Could you check a few things on this model? Use its own coordinates, in mm. A direction names the side the tool comes from. Round coordinates to 2 decimals unless told otherwise and drop trailing zeros. Write each loop counter-clockwise with the first axis right and the second up, starting at its lowest first coordinate (ties: lowest second). Pieces come first, ordered by that corner, then holes. Notation, with made-up numbers: (-14.5, 81) -> (20.5, 81) arc R36 cw to (20.5, 120) -> close; hole circle Ø11 at (80.5, -18.5). An arc over 180 degrees is marked (long way). Answer in a Markdown table with one row per item. Add a question column.
```python
from build123d import *

# Parameters (mm, degrees)
SKETCH1_W           = 31.75
SKETCH1_H           = 3.175
SKETCH1_W_2         = 3.175
SKETCH1_H_2         = 28.575
BOSS_EXTRUDE1_DEPTH = 19.05
SWITCH_MOUNT_REACH  = 5.175
SKETCH2_R           = 1.190625
SKETCH2_W           = 2.54
SKETCH2_H           = 0.254
BRACKET_MOUNT_REACH = 5.175
SKETCH3_R           = 3.175


with BuildPart() as part:
    # Sketch1 → Boss-Extrude1 (new body)
    with BuildSketch(Plane.XY):
        with Locations((-15.875, 1.5875)):
            Rectangle(SKETCH1_W, SKETCH1_H)
        with Locations((-1.5875, -14.2875)):
            Rectangle(SKETCH1_W_2, SKETCH1_H_2)
    extrude(amount=BOSS_EXTRUDE1_DEPTH)

    # Sketch2 → Switch Mount (cut, up to next)
    with BuildSketch(Plane.ZY.offset(3.175), mode=Mode.PRIVATE) as switch_mount_sk1:
        with Locations((4.318, -10.668)):
            Circle(SKETCH2_R)
    switch_mount_tool1 = extrude(switch_mount_sk1.sketch, amount=-SWITCH_MOUNT_REACH, mode=Mode.PRIVATE) & part.part
    add(switch_mount_tool1.solids().sort_by_distance((-3.175, -10.668, 4.318))[0], mode=Mode.SUBTRACT)
    # Sketch2 → Switch Mount (cut, up to next)
    with BuildSketch(Plane.ZY.offset(3.175), mode=Mode.PRIVATE) as switch_mount_sk2:
        with Locations((4.318, -20.193)):
            Circle(SKETCH2_R)
    switch_mount_tool2 = extrude(switch_mount_sk2.sketch, amount=-SWITCH_MOUNT_REACH, mode=Mode.PRIVATE) & part.part
    add(switch_mount_tool2.solids().sort_by_distance((-3.175, -20.193, 4.318))[0], mode=Mode.SUBTRACT)
    # Sketch2 → Switch Mount (cut, up to next)
    with BuildSketch(Plane.ZY.offset(3.175), mode=Mode.PRIVATE) as switch_mount_sk3:
        with Locations((1.27, -25.2222)):
            Rectangle(SKETCH2_W, SKETCH2_H)
    switch_mount_tool3 = extrude(switch_mount_sk3.sketch, amount=-SWITCH_MOUNT_REACH, mode=Mode.PRIVATE) & part.part
    add(switch_mount_tool3.solids().sort_by_distance((-3.175, -25.2222, 1.27))[0], mode=Mode.SUBTRACT)

    # Sketch3 → Bracket Mount (cut, up to next)
    with BuildSketch(Plane.XZ, mode=Mode.PRIVATE) as bracket_mount_sk1:
        with Locations((-9.525, 12.065)):
            Circle(SKETCH3_R)
    bracket_mount_tool1 = extrude(bracket_mount_sk1.sketch, amount=-BRACKET_MOUNT_REACH, mode=Mode.PRIVATE) & part.part
    add(bracket_mount_tool1.solids().sort_by_distance((-9.525, 0, 12.065))[0], mode=Mode.SUBTRACT)
    # Sketch3 → Bracket Mount (cut, up to next)
    with BuildSketch(Plane.XZ, mode=Mode.PRIVATE) as bracket_mount_sk2:
        with Locations((-22.225, 12.065)):
            Circle(SKETCH3_R)
    bracket_mount_tool2 = extrude(bracket_mount_sk2.sketch, amount=-BRACKET_MOUNT_REACH, mode=Mode.PRIVATE) & part.part
    add(bracket_mount_tool2.solids().sort_by_distance((-22.225, 0, 12.065))[0], mode=Mode.SUBTRACT)


solid = part.part
```
(1) I need wall thicknesses on L1, parallel to Y at x = -2, z = 1.5 (3 decimals); L2, parallel to Y at x = -28.5, z = 9.5 (3 decimals); L3, parallel to X at y = -19.5, z = 16.25 (3 decimals). Which ranges of each line are inside material? Lowest first, please.
(2) Suppose I cut it at A-A, the plane z = 2. Please give me the cut outline in (x, y) (3 decimals).
(3) If we mould it in two halves opening along Y, with no side actions, what happens to faces 1 (the face through (-10.1, 0.3, 19.05)), 2 (the face through (-16, 3.175, 9)), 3 (the face through (-2, -25.349, 1)), 4 (the face through (-2, -28.575, 9))? For each: pulls with the +Y half, pulls with the -Y half, needs draft (parallel to the pull), parting line crosses it, or undercut.
(4) On a 3-axis mill with a long thin cutter (end or side, diameter ignored), from which of +Z, -Z, +X, -X, +Y, -Y can I reach the whole of each face in a straight line? I mean faces 5 (the face through (-3.175, -14, 9)), 6 (the face through (-1.61, -21.355, 4.06)), 7 (the face through (-2, -25.095, 1)). Say none if no direction works.
(5) Suppose I cut it at D-D, the plane x = -18. Please give me the cut outline in (y, z) (3 decimals).
(6) Suppose I cut it at C-C, the plane z = 10.25. Please give me the cut outline in (x, y) (3 decimals).
(7) Suppose I cut it at B-B, the plane x = -11. Please give me the cut outline in (y, z) (3 decimals), then the cut area to 3 significant figures.
(8) For P1, Ø1.5, axis at y = -14.5, z = 10, coming from the -X side (3 decimals); P2, Ø7.5, axis at x = -22.225, z = 12.065, coming from the +Y side (3 decimals); P3, Ø4, axis at x = -23, z = 9, coming from the -Y side, each with a flat end and sliding along its axis, tell me the tip position at first contact or that it passes through.
Response:
| question | item | result |
|---|---|---|
| 1 | L1 | -28.575 to -25.349, -25.095 to 3.175 |
| 1 | L2 | 0 to 3.175 |
| 1 | L3 | -3.175 to 0 |
| 2 | outline | (-31.75, 0) -> (-3.175, 0) -> (-3.175, -25.095) -> (0, -25.095) -> (0, 3.175) -> (-31.75, 3.175) -> close; (-3.175, -28.575) -> (0, -28.575) -> (0, -25.349) -> (-3.175, -25.349) -> close |
| 3 | face 1 | needs draft |
| 3 | face 2 | pulls with the +Y half |
| 3 | face 3 | undercut |
| 3 | face 4 | pulls with the -Y half |
| 4 | face 5 | +Z, -Z, -X, -Y |
| 4 | face 6 | +X, -X |
| 4 | face 7 | -Z, +X, -X |
| 5 | outline | (0, 0) -> (3.175, 0) -> (3.175, 19.05) -> (0, 19.05) -> close |
| 6 | outline | (-31.75, 0) -> (-24.83, 0) -> (-24.83, 3.175) -> (-31.75, 3.175) -> close; (-19.62, 0) -> (-12.13, 0) -> (-12.13, 3.175) -> (-19.62, 3.175) -> close; (-6.92, 0) -> (-3.175, 0) -> (-3.175, -28.575) -> (0, -28.575) -> (0, 3.175) -> (-6.92, 3.175) -> close |
| 7 | outline | (0, 0) -> (3.175, 0) -> (3.175, 9.253) -> (0, 9.253) -> close; (0, 14.877) -> (3.175, 14.877) -> (3.175, 19.05) -> (0, 19.05) -> close |
| 7 | area | 42.6 mm² |
| 8 | P1 | x = -3.175 |
| 8 | P2 | y = 3.175 |
| 8 | P3 | y = 0 |
